Read the model definition and answer for the solid it produces. Units are mm, in the model's axes. A direction names the side the tool comes from. Coordinates: 2 decimals unless noted, no trailing zeros. Order: outer loops, then holes, each group sorted by start corner. A loop starts at its lowest first (then second) coordinate and runs counter-clockwise, first axis right, second up. Notation, with made-up numbers: M -36.75,44 L -30.75,44 A14 cw -30.75,58 Z; hole C 20,28.25 d4. An arc over 180 degrees is marked long. Use a Markdown table: item, result. Add a question column.
1) Find section B-B on x = 12.5. Write down the section's boundary in (y, z).
2) This flat-tipped pin is pushed along its axis until it touches: pin 1 Ø1.2 at (x, z) = (43.5, 0) entering from +Y. Where does it stop, or does it pass through?
3) Find section C-C on y = -0.75. Count the separate pieces of the cut face and the enclosed holes in it, plus the area to 3 significant figures.
4) The mould has two halves that part along Z. Classify faces 1 (the face through (38.7, -0.7, -68.2)), 2 (the face through (-38.67, -0.74, 49.1)): released by +Z, released by -Z, zero draft, split by the parting line, or undercut.
5) Find section A-A on z = -63.5. Write down the section's boundary in (x, y), plus the area to 3 significant figures.
6) For faces 3 (the face through (38.6, -0.7, 68.3)), 4 (the face through (-45, -1, 72)), determine the directions among +Z, -Z, +X, -X, +Y, -Y from which every point of the face is accessible in a straight line to the end or side of a thin tool.
7) Find the intervals of material crossed by probe 1 along Z at (x, y) = (7.5, -0.85); probe 2 along X at (y, z) = (-0.15, -8); probe 3 along X at (y, z) = (-0.3, 72), in increasing order. Write a range as [from, to].
from build123d import *

# Parameters (mm, degrees)
F0_W           = 97
F0_H           = 150
F1_DEPTH       = 1.5
F3_D           = 2
F3_CSINK_D     = 4
F3_CSINK_ANGLE = 90
F5_D           = 2


# Not quite as in the source:
# - a feature names something its author has since deleted; it is built from what else it names


with BuildPart() as f1:
    # F0 (on Front) → F1 (new body)
    with BuildSketch(Plane.XZ):
        Rectangle(F0_W, F0_H)
        with BuildLine():
            Line((-4.5249225795, -58.9309873283), (-4.5249225795, -66.1341202259))
            ThreePointArc((-4.5249225795, -66.1341202259), (-5.403602236, -68.2554405695), (-7.5249225795, -69.1341202259))
            Line((-7.5249225795, -69.1341202259), (-36.5249225795, -69.1341202259))
            ThreePointArc((-36.5249225795, -69.1341202259), (-38.6462429231, -68.2554405695), (-39.5249225795, -66.1341202259))
            Line((-39.5249225795, -66.1341202259), (-39.5249225795, -58.9309873283))
            ThreePointArc((-39.5249225795, -58.9309873283), (-38.6462429231, -56.8096669847), (-36.5249225795, -55.9309873283))
            Line((-36.5249225795, -55.9309873283), (-7.5249225795, -55.9309873283))
            ThreePointArc((-7.5249225795, -55.9309873283), (-5.403602236, -56.8096669847), (-4.5249225795, -58.9309873283))
        make_face(mode=Mode.SUBTRACT)
        with BuildLine():
            Line((-36.5249225795, -5), (-7.5249225795, -5))
            ThreePointArc((-7.5249225795, -5), (-5.403602236, -5.8786796564), (-4.5249225795, -8))
            Line((-4.5249225795, -8), (-4.5249225795, -47))
            ThreePointArc((-4.5249225795, -47), (-5.403602236, -49.1213203436), (-7.5249225795, -50))
            Line((-7.5249225795, -50), (-36.5249225795, -50))
            ThreePointArc((-36.5249225795, -50), (-38.6462429231, -49.1213203436), (-39.5249225795, -47))
            Line((-39.5249225795, -47), (-39.5249225795, -8))
            ThreePointArc((-39.5249225795, -8), (-38.6462429231, -5.8786796564), (-36.5249225795, -5))
        make_face(mode=Mode.SUBTRACT)
        with BuildLine():
            ThreePointArc((4.5249225795, -58.9309873283), (5.403602236, -56.8096669847), (7.5249225795, -55.9309873283))
            Line((7.5249225795, -55.9309873283), (36.5249225795, -55.9309873283))
            ThreePointArc((36.5249225795, -55.9309873283), (38.6462429231, -56.8096669847), (39.5249225795, -58.9309873283))
            Line((39.5249225795, -58.9309873283), (39.5249225795, -66.1341202259))
            ThreePointArc((39.5249225795, -66.1341202259), (38.6462429231, -68.2554405695), (36.5249225795, -69.1341202259))
            Line((36.5249225795, -69.1341202259), (7.5249225795, -69.1341202259))
            ThreePointArc((7.5249225795, -69.1341202259), (5.403602236, -68.2554405695), (4.5249225795, -66.1341202259))
            Line((4.5249225795, -66.1341202259), (4.5249225795, -58.9309873283))
        make_face(mode=Mode.SUBTRACT)
        with BuildLine():
            ThreePointArc((39.5249225795, -47), (38.6462429231, -49.1213203436), (36.5249225795, -50))
            Line((36.5249225795, -50), (7.5249225795, -50))
            ThreePointArc((7.5249225795, -50), (5.403602236, -49.1213203436), (4.5249225795, -47))
            Line((4.5249225795, -47), (4.5249225795, -8))
            ThreePointArc((4.5249225795, -8), (5.403602236, -5.8786796564), (7.5249225795, -5))
            Line((7.5249225795, -5), (36.5249225795, -5))
            ThreePointArc((36.5249225795, -5), (38.6462429231, -5.8786796564), (39.5249225795, -8))
            Line((39.5249225795, -8), (39.5249225795, -47))
        make_face(mode=Mode.SUBTRACT)
        with BuildLine():
            ThreePointArc((-4.5249225795, 8), (-5.403602236, 5.8786796564), (-7.5249225795, 5))
            Line((-7.5249225795, 5), (-36.5249225795, 5))
            ThreePointArc((-36.5249225795, 5), (-38.6462429231, 5.8786796564), (-39.5249225795, 8))
            Line((-39.5249225795, 8), (-39.5249225795, 47))
            ThreePointArc((-39.5249225795, 47), (-38.6462429231, 49.1213203436), (-36.5249225795, 50))
            Line((-36.5249225795, 50), (-7.5249225795, 50))
            ThreePointArc((-7.5249225795, 50), (-5.403602236, 49.1213203436), (-4.5249225795, 47))
            Line((-4.5249225795, 47), (-4.5249225795, 8))
        make_face(mode=Mode.SUBTRACT)
        with BuildLine():
            ThreePointArc((-4.5249225795, 58.9309873283), (-5.403602236, 56.8096669847), (-7.5249225795, 55.9309873283))
            Line((-7.5249225795, 55.9309873283), (-36.5249225795, 55.9309873283))
            ThreePointArc((-36.5249225795, 55.9309873283), (-38.6462429231, 56.8096669847), (-39.5249225795, 58.9309873283))
            Line((-39.5249225795, 58.9309873283), (-39.5249225795, 66.1341202259))
            ThreePointArc((-39.5249225795, 66.1341202259), (-38.6462429231, 68.2554405695), (-36.5249225795, 69.1341202259))
            Line((-36.5249225795, 69.1341202259), (-7.5249225795, 69.1341202259))
            ThreePointArc((-7.5249225795, 69.1341202259), (-5.403602236, 68.2554405695), (-4.5249225795, 66.1341202259))
            Line((-4.5249225795, 66.1341202259), (-4.5249225795, 58.9309873283))
        make_face(mode=Mode.SUBTRACT)
        with BuildLine():
            ThreePointArc((7.5249225795, 5), (5.403602236, 5.8786796564), (4.5249225795, 8))
            Line((4.5249225795, 8), (4.5249225795, 47))
            ThreePointArc((4.5249225795, 47), (5.403602236, 49.1213203436), (7.5249225795, 50))
            Line((7.5249225795, 50), (36.5249225795, 50))
            ThreePointArc((36.5249225795, 50), (38.6462429231, 49.1213203436), (39.5249225795, 47))
            Line((39.5249225795, 47), (39.5249225795, 8))
            ThreePointArc((39.5249225795, 8), (38.6462429231, 5.8786796564), (36.5249225795, 5))
            Line((36.5249225795, 5), (7.5249225795, 5))
        make_face(mode=Mode.SUBTRACT)
        with BuildLine():
            Line((7.5249225795, 69.1341202259), (36.5249225795, 69.1341202259))
            ThreePointArc((36.5249225795, 69.1341202259), (38.6462429231, 68.2554405695), (39.5249225795, 66.1341202259))
            Line((39.5249225795, 66.1341202259), (39.5249225795, 58.9309873283))
            ThreePointArc((39.5249225795, 58.9309873283), (38.6462429231, 56.8096669847), (36.5249225795, 55.9309873283))
            Line((36.5249225795, 55.9309873283), (7.5249225795, 55.9309873283))
            ThreePointArc((7.5249225795, 55.9309873283), (5.403602236, 56.8096669847), (4.5249225795, 58.9309873283))
            Line((4.5249225795, 58.9309873283), (4.5249225795, 66.1341202259))
            ThreePointArc((4.5249225795, 66.1341202259), (5.403602236, 68.2554405695), (7.5249225795, 69.1341202259))
        make_face(mode=Mode.SUBTRACT)
    extrude(amount=F1_DEPTH)

    # F3 (through all)
    with Locations(Plane.XZ.offset(1.5)):
        with Locations((-43.5, -72), (43.5, -72), (43.5, 72), (-43.5, 72), (-43.5, 0), (43.5, 0)):
            CounterSinkHole(F3_D / 2, F3_CSINK_D / 2, counter_sink_angle=F3_CSINK_ANGLE)

    # F5 (through all)
    with Locations(Plane.XZ.offset(1.5)):
        with Locations((-37, -72), (0, -72), (37, -72), (0, 52), (-37, 52), (37, 52), (-37, 0), (37, 0)):
            Hole(F5_D / 2)


solid = f1.part
Check result:
| question | item | result |
|---|---|---|
| 1 | outline | M -1.5,-75 L 0,-75 L 0,-69.13 L -1.5,-69.13 Z; M -1.5,-55.93 L 0,-55.93 L 0,-50 L -1.5,-50 Z; M -1.5,-5 L 0,-5 L 0,5 L -1.5,5 Z; M -1.5,50 L 0,50 L 0,55.93 L -1.5,55.93 Z; M -1.5,69.13 L 0,69.13 L 0,75 L -1.5,75 Z |
| 2 | pin 1 | passes through |
| 3 | separate pieces | 1 |
| 3 | enclosed holes | 22 |
| 3 | area | 6,410 mm2 |
| 4 | face 1 | undercut |
| 4 | face 2 | undercut |
| 5 | outline | M -48.5,-1.5 L -39.52,-1.5 L -39.52,0 L -48.5,0 Z; M -4.52,-1.5 L 4.52,-1.5 L 4.52,0 L -4.52,0 Z; M 39.52,-1.5 L 48.5,-1.5 L 48.5,0 L 39.52,0 Z |
| 5 | area | 40.5 mm2 |
| 6 | face 3 | +Y, -Y |
| 6 | face 4 | -Y |
| 7 | probe 1 | z = [-75, -69.13], [-55.93, -50], [-5, 5], [50, 55.93], [69.13, 75] |
| 7 | probe 2 | x = [-48.5, -39.52], [-4.52, 4.52], [39.52, 48.5] |
| 7 | probe 3 | x = [-48.5, -44.5], [-42.5, 42.5], [44.5, 48.5] |
